Input: part model. Units: mm. Frame: model coordinates. A direction names the side the tool comes from. Round coordinates to 2 decimals unless told otherwise and drop trailing zeros. Write each loop counter-clockwise with the first axis right and the second up, starting at its lowest first coordinate (ties: lowest second). Pieces come first, ordered by that corner, then holes. Notation, with made-up numbers: (-26.75, 60) -> (26.25, 60) arc R25 cw to (26.25, 80) -> close; hole circle Ø8 at (13.5, 32). An arc over 180 degrees is marked (long way). Use CSV: the item, a comma, the result in double quotes.
```python
from build123d import *

# Parameters (mm, degrees)
SKETCH1_W            = 30
SKETCH1_H            = 30.8
BOSS_EXTRUDE1_DEPTH  = 7
SKETCH2_R            = 4.15
CUT_EXTRUDE1_DEPTH   = 6.5
SKETCH3_W            = 15
SKETCH3_H            = 1.2
SKETCH3_W_2          = 9
SKETCH3_W_3          = 11
SKETCH3_W_4          = 13
CUT_EXTRUDE2_DEPTH   = 4
SKETCH4_W            = 30
SKETCH4_H            = 3
CUT_EXTRUDE3_DEPTH   = 1.2
SKETCH5_W            = 30
SKETCH5_H            = 3
CUT_EXTRUDE4_DEPTH   = 1.2
SKETCH6_R            = 4.05
CUT_EXTRUDE5_DEPTH   = 27.2
SKETCH7_R            = 4.05
CUT_EXTRUDE6_DEPTH   = 27.2
SKETCH8_R            = 4.75
CUT_EXTRUDE7_DEPTH   = 5
BOSS_EXTRUDE2_DEPTH  = 6.4
FILLET1_R            = 1
BOSS_EXTRUDE3_DEPTH  = 6.4
FILLET2_R            = 1
SKETCH12_W           = 1.5
SKETCH12_H           = 1.344099237
CUT_EXTRUDE8_DEPTH   = 5
SKETCH13_W           = 13
SKETCH13_H           = 7
BOSS_EXTRUDE4_DEPTH  = 1
SKETCH14_W           = 11
SKETCH14_H           = 7
BOSS_EXTRUDE5_DEPTH  = 1
SKETCH15_R           = 2
BOSS_EXTRUDE8_DEPTH  = 5.5
SKETCH16_R           = 2
BOSS_EXTRUDE9_DEPTH  = 5.5
FILLET3_R            = 2
FILLET4_R            = 2
FILLET5_R            = 2
CHAMFER2_SIZE        = 0.5
CHAMFER3_SIZE        = 0.5
SKETCH17_W           = 4
SKETCH17_H           = 7
BOSS_EXTRUDE10_DEPTH = 1.5
FILLET7_R            = 0.5
SKETCH18_R           = 0.9
CUT_EXTRUDE9_DEPTH   = 99.965895754
SKETCH19_R           = 1.6
CUT_EXTRUDE10_DEPTH  = 2
SKETCH20_R           = 0.9
CUT_EXTRUDE11_DEPTH  = 99.965895754
SKETCH21_R           = 1.6
CUT_EXTRUDE12_DEPTH  = 2
CHAMFER6_SIZE        = 0.5
SKETCH22_W           = 6
SKETCH22_H           = 4
BOSS_EXTRUDE11_DEPTH = 0.5
SKETCH23_W           = 6
SKETCH23_H           = 4
BOSS_EXTRUDE12_DEPTH = 0.5


with BuildPart() as part:
    # Sketch1 → Boss-Extrude1 (new body)
    with BuildSketch(Plane(origin=(0, 0, 0), x_dir=(1, 0, 0), z_dir=(0, 1, 0))):
        with Locations((-46.45686042, -50.970505576)):
            Rectangle(SKETCH1_W, SKETCH1_H)
    extrude(amount=BOSS_EXTRUDE1_DEPTH)

    # Sketch2 → Cut-Extrude1 (cut)
    with BuildSketch(Plane.XZ):
        with Locations(Location((-47.47186042, 50.970505576, 0), (0, 0, 270))):
            Circle(SKETCH2_R)
    extrude(amount=-CUT_EXTRUDE1_DEPTH, mode=Mode.SUBTRACT)

    # Sketch3 → Cut-Extrude2 (cut)
    with BuildSketch(Plane.XZ):
        with Locations((-38.95686042, 65.770505576)):
            Rectangle(SKETCH3_W, SKETCH3_H)
        with Locations((-56.95686042, 65.770505576)):
            Rectangle(SKETCH3_W_2, SKETCH3_H)
        with Locations((-36.95686042, 36.170505576)):
            Rectangle(SKETCH3_W_3, SKETCH3_H)
        with Locations((-54.95686042, 36.170505576)):
            Rectangle(SKETCH3_W_4, SKETCH3_H)
    extrude(amount=-CUT_EXTRUDE2_DEPTH, mode=Mode.SUBTRACT)

    # Sketch4 → Cut-Extrude3 (cut)
    with BuildSketch(Plane.XY.offset(66.370505576)):
        with Locations((-46.45686042, 5.5)):
            Rectangle(SKETCH4_W, SKETCH4_H)
    extrude(amount=-CUT_EXTRUDE3_DEPTH, mode=Mode.SUBTRACT)

    # Sketch5 → Cut-Extrude4 (cut)
    with BuildSketch(Plane(origin=(0, 0, 35.570505576), x_dir=(-1, 0, 0), z_dir=(0, 0, -1))):
        with Locations((46.45686042, 5.5)):
            Rectangle(SKETCH5_W, SKETCH5_H)
    extrude(amount=-CUT_EXTRUDE4_DEPTH, mode=Mode.SUBTRACT)

    # Sketch6 → Cut-Extrude5 (cut)
    with BuildSketch(Plane.XY.offset(65.170505576)):
        with Locations((-39.974556342, 7.3)):
            Circle(SKETCH6_R)
    extrude(amount=-CUT_EXTRUDE5_DEPTH, mode=Mode.SUBTRACT)

    # Sketch7 → Cut-Extrude6 (cut)
    with BuildSketch(Plane(origin=(0, 0, 36.770505576), x_dir=(-1, 0, 0), z_dir=(0, 0, -1))):
        with Locations((54.96455223, 7.3)):
            Circle(SKETCH7_R)
    extrude(amount=-CUT_EXTRUDE6_DEPTH, mode=Mode.SUBTRACT)

    # Sketch8 → Cut-Extrude7 (cut)
    with BuildSketch(Plane(origin=(0, 7, 0), x_dir=(1, 0, 0), z_dir=(0, 1, 0))):
        with Locations(Location((-47.47186042, -50.970505576, 0), (0, 0, 270))):
            Circle(SKETCH8_R)
    extrude(amount=-CUT_EXTRUDE7_DEPTH, mode=Mode.SUBTRACT)

    # Sketch10 → Boss-Extrude2 (add)
    with BuildSketch(Plane.XY.offset(65.170505576)):
        Polygon((-31.45686042, 0), (-31.45686042, 7), (-35.85686042, 7), (-35.85686042, 1.7), (-44.45686042, 1.7), (-44.45686042, 0), align=None)
    extrude(amount=BOSS_EXTRUDE2_DEPTH)

    # Fillet1
    fillet1_edges = [part.edges().sort_by_distance(p)[0] for p in [
        (-35.85686042, 1.7, 68.370505576),
    ]]
    fillet(fillet1_edges, radius=FILLET1_R)

    # Sketch11 → Boss-Extrude3 (add)
    with BuildSketch(Plane(origin=(0, 0, 36.770505576), x_dir=(-1, 0, 0), z_dir=(0, 0, -1))):
        Polygon((61.45686042, 7), (61.45686042, 0), (50.45686042, 0), (50.45686042, 1.7), (59.05686042, 1.7), (59.05686042, 7), align=None)
    extrude(amount=BOSS_EXTRUDE3_DEPTH)

    # Fillet2
    fillet2_edges = [part.edges().sort_by_distance(p)[0] for p in [
        (-59.05686042, 1.7, 33.570505576),
    ]]
    fillet(fillet2_edges, radius=FILLET2_R)

    # Sketch12 → Cut-Extrude8 (cut)
    with BuildSketch(Plane(origin=(0, 7, 0), x_dir=(1, 0, 0), z_dir=(0, 1, 0))):
        with Locations((-47.47186042, -56.298455958)):
            Rectangle(SKETCH12_W, SKETCH12_H)
    extrude(amount=-CUT_EXTRUDE8_DEPTH, mode=Mode.SUBTRACT)

    # Sketch13 → Boss-Extrude4 (add)
    with BuildSketch(Plane.XY.offset(71.570505576)):
        with Locations((-37.95686042, 3.5)):
            Rectangle(SKETCH13_W, SKETCH13_H)
    extrude(amount=BOSS_EXTRUDE4_DEPTH)

    # Sketch14 → Boss-Extrude5 (add)
    with BuildSketch(Plane(origin=(0, 0, 30.370505576), x_dir=(-1, 0, 0), z_dir=(0, 0, -1))):
        with Locations((55.95686042, 3.5)):
            Rectangle(SKETCH14_W, SKETCH14_H)
    extrude(amount=BOSS_EXTRUDE5_DEPTH)

    # Sketch15 → Boss-Extrude8 (add)
    with BuildSketch(Plane.XY.offset(71.570505576)):
        with Locations(Location((-36.96455223, 6.8, 0), (0, 0, 174.260829523))):
            Circle(SKETCH15_R)
    extrude(amount=BOSS_EXTRUDE8_DEPTH)

    # Sketch16 → Boss-Extrude9 (add)
    with BuildSketch(Plane(origin=(0, 0, 30.370505576), x_dir=(-1, 0, 0), z_dir=(0, 0, -1))):
        with Locations(Location((57.974556342, 6.8, 0), (0, 0, 174.260829523))):
            Circle(SKETCH16_R)
    extrude(amount=BOSS_EXTRUDE9_DEPTH)

    # Fillet3
    fillet3_edges = [part.edges().sort_by_distance(p)[0] for p in [
        (-59.964531217, 7, 29.870505576),
    ]]
    fillet(fillet3_edges, radius=FILLET3_R)

    # Fillet4
    # the kernel refuses this fillet: 2 mm, written as the material it adds along each edge
    with BuildSketch(Plane(origin=(-55.984581468, 7, 30.370505576), x_dir=(1.0, 6.770411692114482e-12, 0), z_dir=(0, 0, -1))) as fillet4_piece_1:
        with BuildLine():
            CenterArc((1.350683743, -2), FILLET4_R, 90, 56.632987031)
            ThreePointArc((-0.319645565, -0.9), (-0.105311329, -0.469360383), (0, 0))
            Line((0, 0), (1.350683743, 0))
        make_face()
    extrude(amount=1)

    # Fillet5
    # the kernel refuses this fillet: 2 mm, written as the material it adds along each edge
    with BuildSketch(Plane(origin=(-38.954527104, 7, 71.570505576), x_dir=(-1.0, 6.9854393361833605e-12, 0), z_dir=(0, 0, 1)), Plane(origin=(-34.974577356, 7, 72.570505576), x_dir=(1, 0, 0), z_dir=(0, 0, -1))) as fillet5_piece_1:
        with BuildLine():
            CenterArc((1.350683743, -2), FILLET5_R, 90, 56.632987031)
            ThreePointArc((-0.319645565, -0.9), (-0.105311329, -0.469360383), (0, 0))
            Line((0, 0), (1.350683743, 0))
        make_face()
    extrude(amount=1)

    # Chamfer2
    chamfer2_edges = [part.edges().sort_by_distance(p)[0] for p in [
        (-34.974577356, 6.6, 77.070505576),
    ]]
    chamfer(chamfer2_edges, length=CHAMFER2_SIZE)

    # Chamfer3
    chamfer3_edges = [part.edges().sort_by_distance(p)[0] for p in [
        (-59.964531217, 6.6, 24.870505576),
    ]]
    chamfer(chamfer3_edges, length=CHAMFER3_SIZE)

    # Sketch17 → Boss-Extrude10 (add)
    with BuildSketch(Plane(origin=(-31.45686042, 0, 0), x_dir=(0, 0, -1), z_dir=(1, 0, 0))):
        with Locations((-50.570505576, 3.5)):
            Rectangle(SKETCH17_W, SKETCH17_H)
    extrude(amount=BOSS_EXTRUDE10_DEPTH)

    # Fillet7
    fillet7_edges = [part.edges().sort_by_distance(p)[0] for p in [
        (-31.45686042, 3.5, 52.570505576),
        (-31.45686042, 3.5, 48.570505576),
        (-29.95686042, 3.5, 52.570505576),
        (-29.95686042, 3.5, 48.570505576),
    ]]
    fillet(fillet7_edges, radius=FILLET7_R)

    # Sketch18 → Cut-Extrude9 (cut, through all)
    with BuildSketch(Plane.XZ):
        with Locations(Location((-32.45686042, 50.970505576, 0), (0, 0, 270))):
            Circle(SKETCH18_R)
    extrude(amount=-CUT_EXTRUDE9_DEPTH, mode=Mode.SUBTRACT)

    # Sketch19 → Cut-Extrude10 (cut)
    with BuildSketch(Plane.XZ):
        with Locations(Location((-32.45686042, 50.970505576, 0), (0, 0, 270))):
            Circle(SKETCH19_R)
    extrude(amount=-CUT_EXTRUDE10_DEPTH, mode=Mode.SUBTRACT)

    # Sketch20 → Cut-Extrude11 (cut, through all)
    with BuildSketch(Plane.XZ):
        with Locations(Location((-47.45686042, 62.720505576, 0), (0, 0, 270))):
            Circle(SKETCH20_R)
        with Locations(Location((-47.45686042, 39.220505576, 0), (0, 0, 270))):
            Circle(SKETCH20_R)
    extrude(amount=-CUT_EXTRUDE11_DEPTH, mode=Mode.SUBTRACT)

    # Sketch21 → Cut-Extrude12 (cut)
    with BuildSketch(Plane.XZ):
        with Locations(Location((-47.45686042, 62.720505576, 0), (0, 0, 270))):
            Circle(SKETCH21_R)
        with Locations(Location((-47.45686042, 39.220505576, 0), (0, 0, 270))):
            Circle(SKETCH21_R)
    extrude(amount=-CUT_EXTRUDE12_DEPTH, mode=Mode.SUBTRACT)

    # Chamfer6
    # the kernel refuses this chamfer: 0.5 mm, written as the material it takes off along each edge
    with BuildSketch(Plane(origin=(-61.45686042, 0, 28.084664082), x_dir=(1, 0, 0), z_dir=(0, 0, 1))) as chamfer6_piece_1:
        Polygon((CHAMFER6_SIZE, 0), (0, CHAMFER6_SIZE), (0, 0), align=None)
    extrude(amount=38.371682988, mode=Mode.SUBTRACT)
    with BuildSketch(Plane(origin=(-31.45686042, 0, 53.070505576), x_dir=(-1, 0, 0), z_dir=(0, 0, 1))) as chamfer6_piece_2:
        Polygon((CHAMFER6_SIZE, 0), (0, -CHAMFER6_SIZE), (0, 0), align=None)
    extrude(amount=20.785841494, mode=Mode.SUBTRACT)
    with BuildSketch(Plane(origin=(-30.95686042, 0, 52.570505576), x_dir=(0, 0, -1), z_dir=(1, 0, 0))) as chamfer6_piece_3:
        Polygon((CHAMFER6_SIZE, 0), (0, CHAMFER6_SIZE), (0, 0), align=None)
    extrude(amount=0.5, mode=Mode.SUBTRACT)
    with BuildSketch(Plane(origin=(-29.95686042, 0, 49.070505576), x_dir=(-1, 0, 0), z_dir=(0, 0, 1))) as chamfer6_piece_4:
        Polygon((CHAMFER6_SIZE, 0), (0, -CHAMFER6_SIZE), (0, 0), align=None)
    extrude(amount=3, mode=Mode.SUBTRACT)
    with BuildSketch(Plane(origin=(-31.45686042, 0, 35.484664082), x_dir=(-1, 0, 0), z_dir=(0, 0, 1))) as chamfer6_piece_5:
        Polygon((CHAMFER6_SIZE, 0), (0, -CHAMFER6_SIZE), (0, 0), align=None)
    extrude(amount=12.585841494, mode=Mode.SUBTRACT)
    with BuildSketch(Plane(origin=(-30.95686042, 0, 48.570505576), x_dir=(0, 0, 1), z_dir=(1, 0, 0))) as chamfer6_piece_6:
        Polygon((CHAMFER6_SIZE, 0), (0, -CHAMFER6_SIZE), (0, 0), align=None)
    extrude(amount=0.5, mode=Mode.SUBTRACT)
    with BuildSketch(Plane(origin=(-30.95686042, 0, 53.070505576), x_dir=(-1, 0, 0), z_dir=(0, 0, 1))) as chamfer6_piece_7:
        Polygon((0.5 + CHAMFER6_SIZE, 0), (0.5, -CHAMFER6_SIZE), (0.5, 0), align=None)
    revolve(axis=Axis((-30.95686042, 0, 53.070505576), (0, -1, 0)), revolution_arc=90, mode=Mode.SUBTRACT)
    with BuildSketch(Plane(origin=(-30.95686042, 0, 48.070505576), x_dir=(-1, 0, 0), z_dir=(0, 0, -1))) as chamfer6_piece_8:
        Polygon((0.5 + CHAMFER6_SIZE, 0), (0.5, CHAMFER6_SIZE), (0.5, 0), align=None)
    revolve(axis=Axis((-30.95686042, 0, 48.070505576), (0, 1, 0)), revolution_arc=90, mode=Mode.SUBTRACT)
    with BuildSketch(Plane(origin=(-30.45686042, 0, 49.070505576), x_dir=(0, 0, -1), z_dir=(-1, 0, 0))) as chamfer6_piece_9:
        Polygon((0.5 - CHAMFER6_SIZE, 0), (0.5, -CHAMFER6_SIZE), (0.5, 0), align=None)
    revolve(axis=Axis((-30.45686042, 0, 49.070505576), (0, -1, 0)), revolution_arc=90, mode=Mode.SUBTRACT)
    with BuildSketch(Plane(origin=(-30.45686042, 0, 52.070505576), x_dir=(0, 0, 1), z_dir=(-1, 0, 0))) as chamfer6_piece_10:
        Polygon((0.5 - CHAMFER6_SIZE, 0), (0.5, CHAMFER6_SIZE), (0.5, 0), align=None)
    revolve(axis=Axis((-30.45686042, 0, 52.070505576), (0, 1, 0)), revolution_arc=90, mode=Mode.SUBTRACT)

    # Sketch22 → Boss-Extrude11 (add)
    with BuildSketch(Plane(origin=(0, 0, 35.570505576), x_dir=(-1, 0, 0), z_dir=(0, 0, -1))):
        with Locations((45.45686042, 2)):
            Rectangle(SKETCH22_W, SKETCH22_H)
    extrude(amount=BOSS_EXTRUDE11_DEPTH)

    # Sketch23 → Boss-Extrude12 (add)
    with BuildSketch(Plane.XY.offset(66.370505576)):
        with Locations((-49.45686042, 2)):
            Rectangle(SKETCH23_W, SKETCH23_H)
    extrude(amount=BOSS_EXTRUDE12_DEPTH)


solid = part.part
```
Item 1: Section query A-A on z = 70. Return the cut outline in (x, y).
Worked answers:
outline,"(-44.46, 0) -> (-31.96, 0) -> (-31.46, 0.5) -> (-31.46, 7) -> (-35.86, 7) -> (-35.86, 2.7) arc R1 cw to (-36.86, 1.7) -> (-44.46, 1.7) -> close"
Item 2: Line query: line 1 (X direction, y = 5.75, z = 59); line 2 (Z direction, x = -56.5, y = 2); line 3 (Z direction, x = -44, y = 3). Output: solid intervals per line, ascending.
Worked answers:
line 1,"x = -61.46 to -58.71, -51.22 to -43.72, -36.23 to -31.46"
line 2,"z = 29.37 to 30.37, 36.77 to 65.17"
line 3,"z = 35.07 to 47.73, 54.21 to 65.17, 71.57 to 72.57"
Item 3: Section query B-B on x = -41. Return the cut outline in (y, z), plus the area to 3 significant figures.
Worked answers:
outline,"(0, 36.77) -> (7, 36.77) -> (7, 37.97) -> (3.38, 37.97) -> (3.38, 65.17) -> (1.7, 65.17) -> (1.7, 71.57) -> (7, 71.57) -> (7, 72.57) -> (0, 72.57) -> close"
area,"118 mm²"
Item 4: Set-up query: faces 5 (the face through (-53, 7, 30)), 6 (the face through (-47, 2, 38)), 7 (the face through (-46.457, 2, 66)), 8 (the face through (-47, 5, 56.971)). Return all of +Z, -Z, +X, -X, +Y, -Y with unobstructed straight access to the full face (end or side cutting, diameter ignored); none if empty.
Worked answers:
face 5,"+Z, -Z, +X, +Y"
face 6,"-Y"
face 7,"+Z, +Y, -Y"
face 8,"+Y"
Item 5: Pull-direction query (Z, two-part tool) for faces 1 (the face through (-48.222, 5, 56)), 2 (the face through (-48.457, 2, 36)), 3 (the face through (-38, 3, 72.571)), 4 (the face through (-55, 6, 63.971)); classes: +Z half, -Z half, draft (parallel to the pull), parting line (faces both ways), or undercut.
Worked answers:
face 1,"undercut"
face 2,"draft"
face 3,"+Z half"
face 4,"undercut"
Item 6: First-contact query: pin 1 Ø3 at (x, z) = (-47.46, 39.22) entering from -Y; pin 2 Ø7.5 at (x, z) = (-47.47, 50.97) entering from -Y; pin 3 Ø3.5 at (x, y) = (-41.5, 4) entering from -Z; pin 4 Ø7 at (x, z) = (-41.5, 69.5) entering from +Y. Flat tips, straight axial feed; report the tip coordinate or a pass-through.
Worked answers:
pin 1,"stops at y = 2"
pin 2,"passes through"
pin 3,"stops at z = 35.07"
pin 4,"stops at y = 7.84"
